from build123d import *

# Parameters (mm, degrees)
SKETCH1_W           = 206
SKETCH1_H           = 81
SKETCH1_R           = 2
SKETCH1_R_2         = 11
SKETCH1_W_2         = 5
SKETCH1_H_2         = 5
BOSS_EXTRUDE4_DEPTH = 5
FILLET9_R           = 5


with BuildPart() as part:
    # Sketch1 → Boss-Extrude4 (new body)
    with BuildSketch(Plane(origin=(0, 0, 0), x_dir=(1, 0, 0), z_dir=(0, 1, 0))):
        with Locations((5.102707087, 13.156325227)):
            Rectangle(SKETCH1_W, SKETCH1_H)
        with Locations(Location((-54.897292913, 48.156325227, 0), (0, 0, 270))):
            Circle(SKETCH1_R, mode=Mode.SUBTRACT)
        with Locations(Location((-54.897292913, -21.843674773, 0), (0, 0, 90))):
            Circle(SKETCH1_R, mode=Mode.SUBTRACT)
        with Locations(Location((65.102707087, -21.843674773, 0), (0, 0, 270))):
            Circle(SKETCH1_R, mode=Mode.SUBTRACT)
        with Locations(Location((65.102707087, 48.156325227, 0), (0, 0, 90))):
            Circle(SKETCH1_R, mode=Mode.SUBTRACT)
        with Locations(Location((-48.397292913, 13.156325227, 0), (0, 0, 270))):
            Circle(SKETCH1_R, mode=Mode.SUBTRACT)
        with Locations(Location((58.602707087, 13.156325227, 0), (0, 0, 90))):
            Circle(SKETCH1_R, mode=Mode.SUBTRACT)
        with Locations(Location((-74.397292913, 13.156325227, 0), (0, 0, 270))):
            Circle(SKETCH1_R_2, mode=Mode.SUBTRACT)
        with Locations((57.602707087, 48.156325227)):
            Rectangle(SKETCH1_W_2, SKETCH1_H_2, mode=Mode.SUBTRACT)
        with Locations((-62.397292913, 48.156325227)):
            Rectangle(SKETCH1_W_2, SKETCH1_H_2, mode=Mode.SUBTRACT)
        with Locations((-47.397292913, 48.156325227)):
            Rectangle(SKETCH1_W_2, SKETCH1_H_2, mode=Mode.SUBTRACT)
        with Locations((72.602707087, 48.156325227)):
            Rectangle(SKETCH1_W_2, SKETCH1_H_2, mode=Mode.SUBTRACT)
        with Locations((72.602707087, -21.843674773)):
            Rectangle(SKETCH1_W_2, SKETCH1_H_2, mode=Mode.SUBTRACT)
        with Locations((57.602707087, -21.843674773)):
            Rectangle(SKETCH1_W_2, SKETCH1_H_2, mode=Mode.SUBTRACT)
        with Locations((-47.397292913, -21.843674773)):
            Rectangle(SKETCH1_W_2, SKETCH1_H_2, mode=Mode.SUBTRACT)
        with Locations((-62.397292913, -21.843674773)):
            Rectangle(SKETCH1_W_2, SKETCH1_H_2, mode=Mode.SUBTRACT)
        with Locations((-48.397292913, 20.656325227)):
            Rectangle(SKETCH1_W_2, SKETCH1_H_2, mode=Mode.SUBTRACT)
        with Locations((-48.397292913, 5.656325227)):
            Rectangle(SKETCH1_W_2, SKETCH1_H_2, mode=Mode.SUBTRACT)
        with Locations((58.602707087, 5.656325227)):
            Rectangle(SKETCH1_W_2, SKETCH1_H_2, mode=Mode.SUBTRACT)
        with Locations((58.602707087, 20.656325227)):
            Rectangle(SKETCH1_W_2, SKETCH1_H_2, mode=Mode.SUBTRACT)
    extrude(amount=BOSS_EXTRUDE4_DEPTH)

    # Fillet9
    fillet9_edges = [part.edges().sort_by_distance(p)[0] for p in [
        (-97.897292913, 2.5, -53.656325227),
        (108.102707087, 2.5, -53.656325227),
        (108.102707087, 2.5, 27.343674773),
        (-97.897292913, 2.5, 27.343674773),
    ]]
    fillet(fillet9_edges, radius=FILLET9_R)


solid = part.part
Read the model definition and answer for the solid it produces. Units are mm, in the model's axes. A direction names the side the tool comes from. Coordinates: 2 decimals unless noted, no trailing zeros. Loops run counter-clockwise (first coordinate to the right, second up) from the corner with the lowest first, then second, coordinate; pieces in that order, holes last.
Q1. The part is cut by section A-A on z = -21. Write down the section's boundary in (x, y).
Q2. The mould has two halves that part along X. Classify faces 1 (the face through (-48, 2, -8.156)), 2 (the face through (4, 2, -53.656)), 3 (the face through (-96.471, 2.535, -52.153)): +X half, -X half, draft (parallel to the pull), parting line (faces both ways), or undercut.
Q3. The part is cut by section C-C on y = 4.2. Give the number of separate pieces and of enclosed holes in the cut face, and give its area (3 significant figures).
Q4. Consider probe 1 along Z at (x, y) = (-45.5, 3.8); probe 2 along Z at (x, y) = (-50.5, 1.4); probe 3 along Z at (x, y) = (-75, 2.85). Determine where each line is inside the solid, lowest interval first.
Q5. Which of the six approach directions +Z, -Z, +X, -X, +Y, -Y give full straight-line access (tool end or side, diameter ignored) to faces 4 (the face through (70.103, 2, -48)), 5 (the face through (106.599, 2.535, 25.918))?
Q6. The part is cut by section B-B on x = -77. Write down the section's boundary in (y, z), and give its area (3 significant figures).
Results below:
1. outline: (-97.9, 0) - (-82.11, 0) - (-82.11, 5) - (-97.9, 5) - close; (-66.69, 0) - (-50.9, 0) - (-50.9, 5) - (-66.69, 5) - close; (-45.9, 0) - (56.1, 0) - (56.1, 5) - (-45.9, 5) - close; (61.1, 0) - (108.1, 0) - (108.1, 5) - (61.1, 5) - close
2. face 1: undercut
2. face 2: draft
2. face 3: -X half
3. separate pieces: 1
3. enclosed holes: 19
3. area: 15,900 mm2
4. probe 1: z = -53.66 to -50.66, -45.66 to 19.34, 24.34 to 27.34
4. probe 2: z = -53.66 to -23.16, -18.16 to -8.16, -3.16 to 27.34
4. probe 3: z = -53.66 to -24.14, -2.17 to 27.34
5. face 4: +Y, -Y
5. face 5: +Z, +X, +Y, -Y
6. outline: (0, -53.66) - (5, -53.66) - (5, -23.84) - (0, -23.84) - close; (0, -2.47) - (5, -2.47) - (5, 27.34) - (0, 27.34) - close
6. area: 298 mm2
